The listing builds one solid part. Answer for the finished solid, in the listing's coordinates (mm). Round coordinates to 2 decimals unless told otherwise and drop trailing zeros. Order: outer loops, then holes, each group sorted by start corner. A loop starts at its lowest first (then second) coordinate and runs counter-clockwise, first axis right, second up. Notation, with made-up numbers: (58, 27.5) -> (90, 27.5) arc R18 cw to (90, 35.5) -> close; hole circle Ø4 at (29.5, -31). An arc over 180 degrees is marked (long way). Answer in a Markdown table with one row per item. Add a question column.
```python
from build123d import *

# Parameters (mm, degrees)
BOSS_EXTRUDE1_DEPTH = 3
TAPPED_HOLE1_D      = 5


with BuildPart() as part:
    # Sketch1 → Boss-Extrude1 (new body)
    with BuildSketch(Plane(origin=(0, 0, 0), x_dir=(0, 0, -1), z_dir=(1, 0, 0))):
        Polygon((5.773502692, 0), (2.886751346, 5), (-2.886751346, 5), (-5.773502692, 0), (-2.886751346, -5), (2.886751346, -5), align=None)
    extrude(amount=BOSS_EXTRUDE1_DEPTH)

    # Tapped Hole1 (through all)
    with Locations(Plane.ZY):
        with Locations((0, 0)):
            Hole(TAPPED_HOLE1_D / 2)

    # Sketch6 → Cut-Revolve1 (revolve, cut)
    with BuildSketch(Plane(origin=(0, 0, 0), x_dir=(1, 0, 0), z_dir=(0, 1, 0))):
        Polygon((0, 5), (0.446581987, 5.773502692), (0, 5.773502692), align=None)
    cut_revolve1 = revolve(axis=Axis((0, 0, 0), (1, 0, 0)), mode=Mode.SUBTRACT)

    # Mirror1: Cut-Revolve1 across plane
    add(cut_revolve1.mirror(Plane.ZY.offset(-1.5)), mode=Mode.SUBTRACT)


solid = part.part
```
Item 1: Find the intervals of material crossed by probe 1 along Y at (x, z) = (1.7, 0.25); probe 2 along Y at (x, z) = (1.75, 1.75); probe 3 along Z at (x, y) = (2.2, 1.75), in increasing order. Write a range as [from, to].
Item 2: For a pull along Z with two mould halves and no side action, classify faces 1 (the face through (1, 5, 0)), 2 (the face through (1.52, -2.44, 0.54)), 3 (the face through (1.479, -2.535, -4.31)), 4 (the face through (1.479, -2.465, 4.35)) as released by +Z, released by -Z, zero draft, split by the parting line, or undercut.
Item 3: The part is cut by section A-A, the plane x = 0.8. Give the vertices of the cut face in (y, z).
Item 4: A flat-ended cylindrical pin translates along its axis: P1, Ø1.5, axis at x = 1.5, y = 3.5, coming from the -Z side. Find the tip coordinate at first contact, or state that the pin passes through.
Resolved:
| question | item | result |
|---|---|---|
| 1 | probe 1 | [-5, -2.49], [2.49, 5] |
| 1 | probe 2 | [-5, -1.79], [1.79, 5] |
| 1 | probe 3 | [-4.76, -1.79], [1.79, 4.76] |
| 2 | face 1 | zero draft |
| 2 | face 2 | undercut |
| 2 | face 3 | released by -Z |
| 2 | face 4 | released by +Z |
| 3 | outline | (-5, -2.89) -> (0, -5.77) -> (5, -2.89) -> (5, 2.89) -> (0, 5.77) -> (-5, 2.89) -> close; hole circle Ø5 at (0, 0) |
| 4 | P1 | z = -4.19 |
